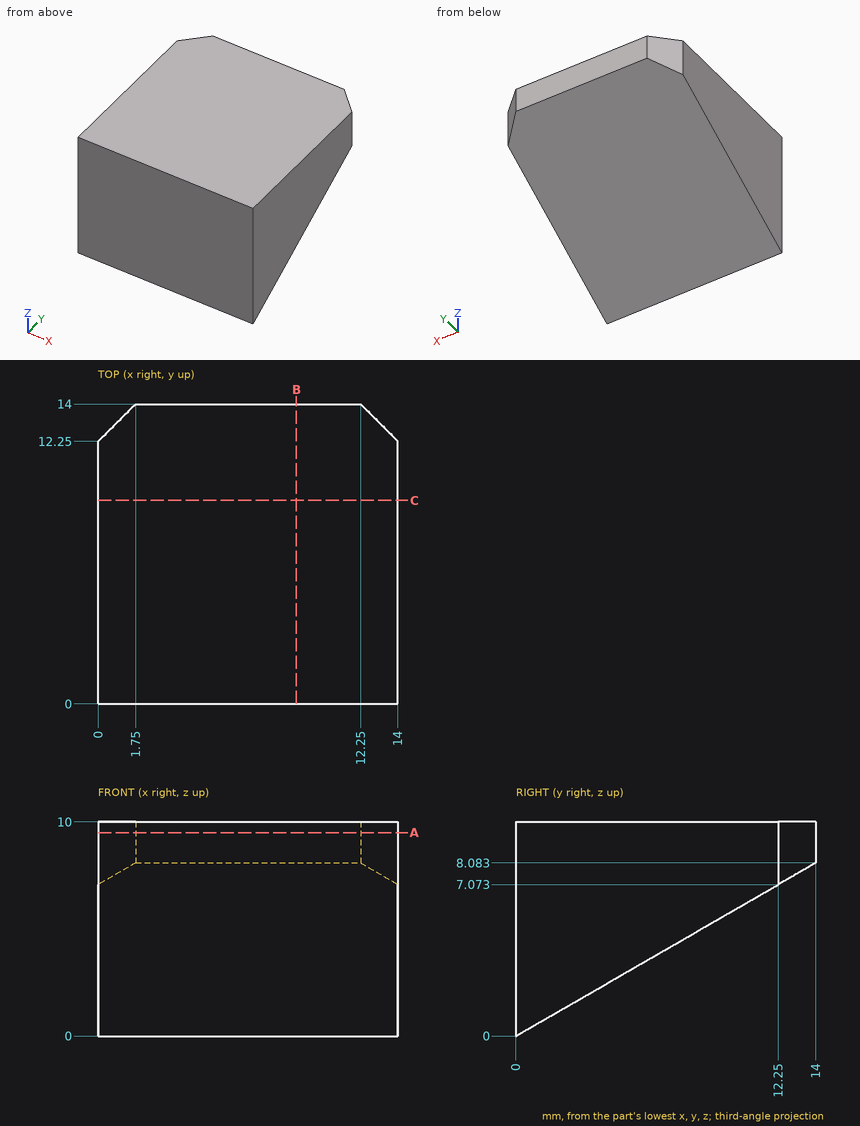
Part print with two shaded views. Sizes in mm from the minimum x, y, z corner. Round coordinates to 2 decimals unless told otherwise and drop trailing zeros. Write each loop counter-clockwise with the first axis right and the second up, starting at its lowest first coordinate (ties: lowest second). Pieces come first, ordered by that corner, then holes. Notation, with made-up numbers: M 60,25.25 L 109,25.25 A25 cw 109,49.25 Z; hole C -23,1.25 d6. An arc over 180 degrees is marked long. Put each result on its own line as item: value. Start each with the question number.
1) Saw through at A-A, the plane z = 9.5. Write the cut outline in (x, y), and give its area (3 significant figures).
2) Saw through at C-C, the plane y = 9.5. Write the cut outline in (x, z) (1 decimal).
3) Drill centre lines: probe 1 along Z at (x, y) = (10.25, 12.25); probe 2 along Z at (x, y) = (9.25, 3.75) (1 decimal); probe 3 along Y at (x, z) = (12.5, 6.75) (1 decimal). Where is each one in solid material? Low to high. Write a range as [from, to].
4) Saw through at B-B, the plane x = 9.25. Write the cut outline in (y, z).
Resolved:
1. outline: M 0,0 L 14,0 L 14,12.25 L 12.25,14 L 1.75,14 L 0,12.25 Z
1. area: 193 mm²
2. outline: M 0,5.5 L 14,5.5 L 14,10 L 0,10 Z
3. probe 1: [7.07, 10]
3. probe 2: [2.2, 10]
3. probe 3: [0, 11.7]
4. outline: M 0,0 L 14,8.08 L 14,10 L 0,10 Z
